Drawing for the job (mm, zero at the part's lowest x, y, z). A direction names the side the tool comes from. Round coordinates to 2 decimals unless told otherwise and drop trailing zeros. Order: outer loops, then holes, each group sorted by start corner. A loop starts at its lowest first (then second) coordinate and runs counter-clockwise, first axis right, second up. Notation, with made-up numbers: (71, 72) - (108, 72) arc R27 cw to (108, 96) - close; hole circle Ø6 at (38, 46). An arc over 180 degrees is marked (long way). Answer as a JSON object with one key per item and string values.
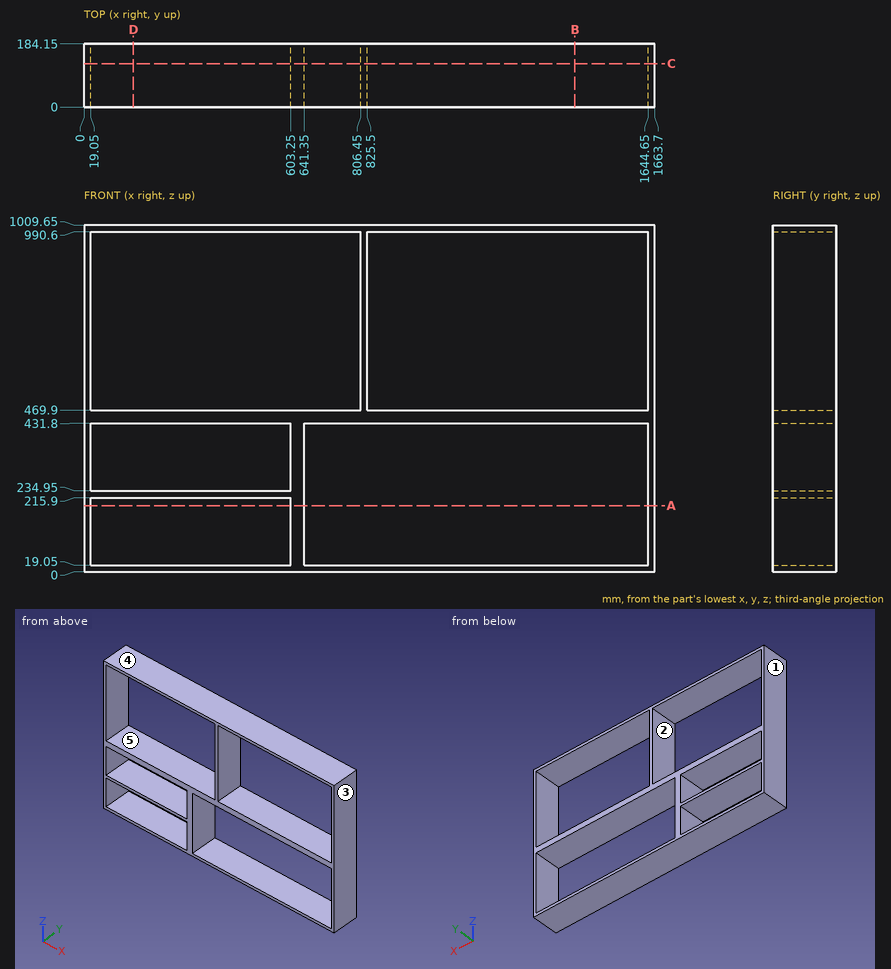
Item 1: Cut at C-C (y = 127). Write the cut outline in (x, z).
Taken from the geometry:
{"outline": "(0, 0) - (1663.7, 0) - (1663.7, 1009.65) - (0, 1009.65) - close; hole (19.05, 19.05) - (603.25, 19.05) - (603.25, 215.9) - (19.05, 215.9) - close; hole (19.05, 234.95) - (603.25, 234.95) - (603.25, 431.8) - (19.05, 431.8) - close; hole (19.05, 469.9) - (806.45, 469.9) - (806.45, 990.6) - (19.05, 990.6) - close; hole (641.35, 19.05) - (1644.65, 19.05) - (1644.65, 431.8) - (641.35, 431.8) - close; hole (825.5, 469.9) - (1644.65, 469.9) - (1644.65, 990.6) - (825.5, 990.6) - close"}
Item 2: Cut at A-A (z = 192). Write the cut outline in (x, y), plus the area to 3 significant figures.
Taken from the geometry:
{"outline": "(0, 0) - (19.05, 0) - (19.05, 184.15) - (0, 184.15) - close; (603.25, 0) - (641.35, 0) - (641.35, 184.15) - (603.25, 184.15) - close; (1644.65, 0) - (1663.7, 0) - (1663.7, 184.15) - (1644.65, 184.15) - close", "area": "14,000 mm2"}
Item 3: Tool access for the marked faces 1 and 2: list every direction of +Z, -Z, +X, -X, +Y, -Y with a clear straight run to the whole face (end or side of a thin tool).
Taken from the geometry:
{"face 1": "+Z, -Z, -X, +Y, -Y", "face 2": "+Y, -Y"}
Item 4: Probe L1, parallel to Z at x = 1442.5, y = 146; L2, parallel to X at y = 48, z = 238.5; L3, parallel to Z at x = 138, y = 35. List the from-to ranges inside material, lowest first. Write a range as from..to.
Taken from the geometry:
{"L1": "0..19.05, 431.8..469.9, 990.6..1009.65", "L2": "0..19.05, 603.25..641.35, 1644.65..1663.7", "L3": "0..19.05, 215.9..234.95, 431.8..469.9, 990.6..1009.65"}
Item 5: Cut at D-D (x = 144). Write the cut outline in (y, z).
Taken from the geometry:
{"outline": "(0, 0) - (184.15, 0) - (184.15, 19.05) - (0, 19.05) - close; (0, 215.9) - (184.15, 215.9) - (184.15, 234.95) - (0, 234.95) - close; (0, 431.8) - (184.15, 431.8) - (184.15, 469.9) - (0, 469.9) - close; (0, 990.6) - (184.15, 990.6) - (184.15, 1009.65) - (0, 1009.65) - close"}
Item 6: Cut at B-B (x = 1430.5). Write the cut outline in (y, z), plus the area to 3 significant figures.
Taken from the geometry:
{"outline": "(0, 0) - (184.15, 0) - (184.15, 19.05) - (0, 19.05) - close; (0, 431.8) - (184.15, 431.8) - (184.15, 469.9) - (0, 469.9) - close; (0, 990.6) - (184.15, 990.6) - (184.15, 1009.65) - (0, 1009.65) - close", "area": "14,000 mm2"}
Item 7: Drop a flat-ended pin along its axis: P1, Ø6, axis at x = 207, y = 86, coming from the -Z side. Give the stop position or say it passes through.
Taken from the geometry:
{"P1": "z = 0"}
Item 8: Two-plate mould, pull along X, no slides. Class the marked faces 3, 4 and 5: pulls with the +X half, pulls with the -X half, needs draft (parallel to the pull), parting line crosses it, or undercut.
Taken from the geometry:
{"face 3": "pulls with the +X half", "face 4": "needs draft", "face 5": "undercut"}
